from build123d import *

# Parameters (mm, degrees)
SKETCH1_W           = 50
SKETCH1_H           = 52
SKETCH1_R           = 9
SKETCH1_R_2         = 2
BOSS_EXTRUDE1_DEPTH = 2.75
SKETCH2_W           = 50
SKETCH2_H           = 2.75
BOSS_EXTRUDE2_DEPTH = 52
CUT_EXTRUDE1_DEPTH  = 78.672388917


with BuildPart() as part:
    # Sketch1 → Boss-Extrude1 (new body)
    with BuildSketch(Plane(origin=(0, 0, 0), x_dir=(1, 0, 0), z_dir=(0, 1, 0))):
        Rectangle(SKETCH1_W, SKETCH1_H)
        with Locations(Location((0, 0, 0), (0, 0, 270))):
            Circle(SKETCH1_R, mode=Mode.SUBTRACT)
        with Locations(Location((-14.5, 0, 0), (0, 0, 270))):
            Circle(SKETCH1_R_2, mode=Mode.SUBTRACT)
        with Locations(Location((14.5, 0, 0), (0, 0, 270))):
            Circle(SKETCH1_R_2, mode=Mode.SUBTRACT)
    extrude(amount=BOSS_EXTRUDE1_DEPTH)

    # Sketch2 → Boss-Extrude2 (add)
    with BuildSketch(Plane(origin=(0, 0, 0), x_dir=(1, 0, 0), z_dir=(0, 1, 0))):
        with Locations((0, -24.625)):
            Rectangle(SKETCH2_W, SKETCH2_H)
    extrude(amount=BOSS_EXTRUDE2_DEPTH)

    # Sketch4 → Cut-Extrude1 (cut, through all)
    with BuildSketch(Plane.XY.offset(26)):
        with BuildLine():
            Line((-14, 14), (-8, 14))
            ThreePointArc((-8, 14), (-6, 12), (-8, 10))
            Line((-8, 10), (-14, 10))
            ThreePointArc((-14, 10), (-16, 12), (-14, 14))
        make_face()
        with BuildLine():
            Line((8, 14), (14, 14))
            ThreePointArc((14, 14), (16, 12), (14, 10))
            Line((14, 10), (8, 10))
            ThreePointArc((8, 10), (6, 12), (8, 14))
        make_face()
        with BuildLine():
            Line((8, 42), (14, 42))
            ThreePointArc((14, 42), (16, 40), (14, 38))
            Line((14, 38), (8, 38))
            ThreePointArc((8, 38), (6, 40), (8, 42))
        make_face()
        with BuildLine():
            Line((-14, 42), (-8, 42))
            ThreePointArc((-8, 42), (-6, 40), (-8, 38))
            Line((-8, 38), (-14, 38))
            ThreePointArc((-14, 38), (-16, 40), (-14, 42))
        make_face()
    extrude(amount=-CUT_EXTRUDE1_DEPTH, mode=Mode.SUBTRACT)


solid = part.part
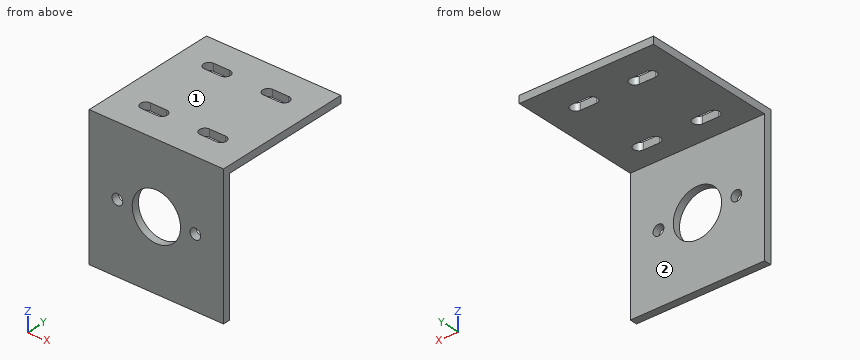
Geometry: final body of the model. Coordinates: model frame, mm. Face numbers are marked on the shaded views. A direction names the side the tool comes from. Give positions to 0.01 mm unless a question says otherwise; leave off trailing zeros. Order: outer loops, then holes, each group sorted by start corner. A loop starts at its lowest first (then second) coordinate and runs counter-clockwise, first axis right, second up. Notation, with made-up numbers: (-26.75, 12) -> (-8.75, 12) arc R30 ccw to (-8.75, 37) -> close; hole circle Ø4 at (-9.5, 80). An arc over 180 degrees is marked (long way). Answer as a JSON object with one key per item and string values.
Q1. First-contact query: pin 1 (5 mm diameter, centred on x = -14.5, z = 0, fed in from +Y); pin 2 (12 mm diameter, centred on x = 12, y = 26, fed in from -Z); pin 3 (2.5 mm diameter, centred on x = 14.5, z = 0, fed in from +Y). Flat tips, straight axial feed; report the tip coordinate or a pass-through.
Entries:
{"pin 1": "stops at y = 2.75", "pin 2": "stops at z = 23.25", "pin 3": "passes through"}
Q2. Section A-A (y = 12). Output: boundary loops of the cut face in (x, z).
Entries:
{"outline": "(-25, 23.25) -> (-16, 23.25) -> (-16, 26) -> (-25, 26) -> close; (-6, 23.25) -> (6, 23.25) -> (6, 26) -> (-6, 26) -> close; (16, 23.25) -> (25, 23.25) -> (25, 26) -> (16, 26) -> close"}
Q3. Section B-B (z = -3.5). Output: boundary loops of the cut face in (x, y).
Entries:
{"outline": "(-25, 0) -> (-8.29, 0) -> (-8.29, 2.75) -> (-25, 2.75) -> close; (8.29, 0) -> (25, 0) -> (25, 2.75) -> (8.29, 2.75) -> close"}
Q4. Access query for the marked faces 1 and 2. Directions: +Z, -Z, +X, -X, +Y, -Y. A direction counts if a zero-diameter tool reaches every point of the face in a straight line with its end or side. Return the directions, or none.
Entries:
{"face 1": "+Z, +X, -X, +Y, -Y", "face 2": "-Z, +X, -X, +Y"}
Q5. Section C-C (x = 18.5). Output: boundary loops of the cut face in (y, z).
Entries:
{"outline": "(0, -26) -> (2.75, -26) -> (2.75, 23.25) -> (52, 23.25) -> (52, 26) -> (0, 26) -> close"}
Q6. Material intervals for probe 1 along X at (y, z) = (1.05, 0); probe 2 along Y at (x, z) = (19, -23); probe 3 along Z at (x, y) = (-3.5, 7.5), sorted ascending.
Entries:
{"probe 1": "x = -25 to -16.5, -12.5 to -9, 9 to 12.5, 16.5 to 25", "probe 2": "y = 0 to 2.75", "probe 3": "z = 23.25 to 26"}
Q7. Section D-D (z = -13). Output: boundary loops of the cut face in (x, y), plus the area to 4 significant figures.
Entries:
{"outline": "(-25, 0) -> (25, 0) -> (25, 2.75) -> (-25, 2.75) -> close", "area": "137.5 mm^2"}
